Geometry: final body of the model. Coordinates: model frame, mm. A direction names the side the tool comes from. Give positions to 0.01 mm unless a question says otherwise; leave off trailing zeros.
```python
from build123d import *

# Parameters (mm, degrees)
BOSS_EXTRUDE1_DEPTH       = 2
M5X0_8_TAPPED_HOLE1_D     = 4.2
M5X0_8_TAPPED_HOLE1_DEPTH = 5
M5X0_8_TAPPED_HOLE1_TIP   = 1.2618073


with BuildPart() as part:
    # Sketch1 → Boss-Extrude1 (new body)
    with BuildSketch(Plane(origin=(0, 0, 0), x_dir=(1, 0, 0), z_dir=(0, 1, 0))):
        Polygon((2.886751346, 5), (-2.886751346, 5), (-5.773502692, 0), (-2.886751346, -5), (2.886751346, -5), (5.773502692, 0), align=None)
    extrude(amount=BOSS_EXTRUDE1_DEPTH)

    # Sketch2 → Revolve1 (revolve)
    with BuildSketch(Plane.XY):
        with BuildLine():
            Line((4.75, 2), (0, 2))
            Line((0, 2), (0, 11))
            add(Edge.make_bspline(
                [(0, 11), (0.622499022, 11), (4.75, 8.004236855), (4.75, 2)],
                knots=[0, 0, 0, 0, 1, 1, 1, 1], degree=3))
        make_face()
    revolve(axis=Axis((0, 11, 0), (0, -1, 0)))

    # M5x0.8 Tapped Hole1
    with Locations(Plane(origin=(0, 0, 0), x_dir=(-1, 0, 0), z_dir=(0, -1, 0))):
        with Locations((0, 0)):
            Hole(M5X0_8_TAPPED_HOLE1_D / 2, depth=M5X0_8_TAPPED_HOLE1_DEPTH)
            with Locations((0, 0, -(M5X0_8_TAPPED_HOLE1_DEPTH + M5X0_8_TAPPED_HOLE1_TIP / 2))):  # 118° drill point
                Cone(0, M5X0_8_TAPPED_HOLE1_D / 2, M5X0_8_TAPPED_HOLE1_TIP, mode=Mode.SUBTRACT)


solid = part.part
```
Item 1: Pin query (flat end, axial travel): pin 1 Ø6 at (x, y) = (-3.5, 7.5) entering from -Z; pin 2 Ø6 at (y, z) = (8, -3.5) entering from -X; pin 3 Ø2 at (y, z) = (3.5, -1.5) entering from -X. Return the tip coordinate at first contact, or that it passes through.
Found:
pin 1: stops at z = -4.05
pin 2: stops at x = -3.88
pin 3: stops at x = -4.67
Item 2: Reachability of faces 4 (the face through (2.003, 2.535, -0.631)), 5 (the face through (4.31, 0.986, 2.535)) from +Z, -Z, +X, -X, +Y, -Y: full face, straight path, thin tool, end or side. Return the list, or none.
Found:
face 4: -Y
face 5: +Z, +X, +Y, -Y
Item 3: Line query: L1, parallel to Z at x = 0, y = 2.3; L2, parallel to Z at x = 0, y = 1.35; L3, parallel to Y at x = 3, z = 4. Output: solid intervals per line, ascending.
Found:
L1: z = -4.75 to -2.1, 2.1 to 4.75
L2: z = -5 to -2.1, 2.1 to 5
L3: y = 0 to 2
Item 4: Pull-direction query (Z, two-part tool) for faces 1 (the face through (-0.34, 6.04, 0.14)), 2 (the face through (5, 2, 1)), 3 (the face through (0, 1, 5)); classes: +Z half, -Z half, draft (parallel to the pull), parting line (faces both ways), or undercut.
Found:
face 1: undercut
face 2: draft
face 3: +Z half
